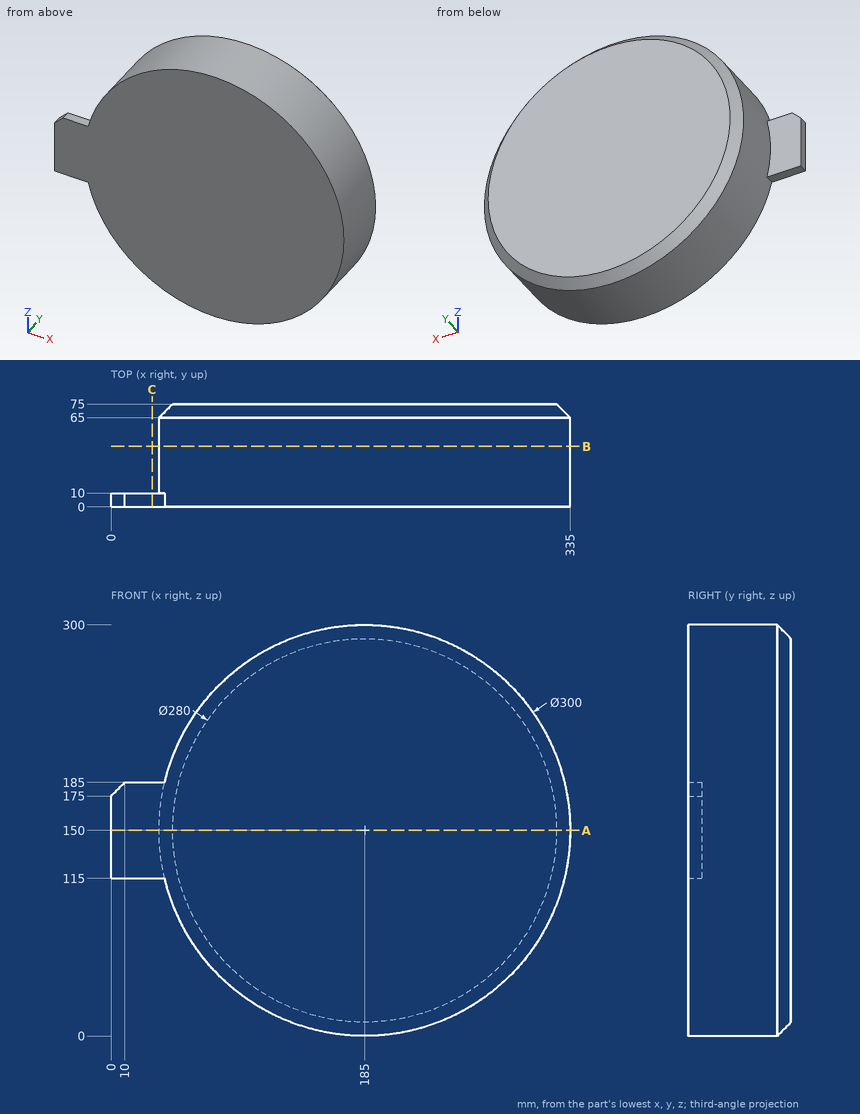
Could you check a few things on this drawing? It's one solid part, dimensions in mm from its lowest x, y, z. Round coordinates to 2 decimals unless told otherwise and drop trailing zeros. Write each loop counter-clockwise with the first axis right and the second up, starting at its lowest first coordinate (ties: lowest second). Pieces come first, ordered by that corner, then holes. Notation, with made-up numbers: (-5, -9) -> (27, -9) arc R20 ccw to (27, 21) -> close; hole circle Ø1 at (-18.5, 47.25). An arc over 180 degrees is marked (long way). Use one line per item in the form item = value. Start each with the question number.
Q1. If I drill on probe 1 along Y at (x, z) = (17, 139); probe 2 along X at (y, z) = (67.5, 143); probe 3 along Z at (x, y) = (68, 34.5), over which ranges is the centre line in solid material (lowest first)? Write a range as [from, to].
Q2. Imagine slicing it at A-A (z = 150). Please give me the cut outline in (x, y).
Q3. I'm going to push flat-ended pins straight in: P1, Ø4, axis at x = 86.5, y = 52.5, coming from the +Z side; P2, Ø6, axis at y = 21, z = 191, coming from the +X side; P3, Ø19.5, axis at x = 15, z = 148, coming from the +Y side. Where does each tip first touch, or does it pass through?
Q4. Imagine slicing it at C-C (x = 30). Please give me the cut outline in (y, z), then the cut area to 3 significant figures.
Q5. Imagine slicing it at B-B (y = 44). Please give me the cut outline in (x, z), then the cut area to 3 significant figures.
Worked out:
q1.probe_1 = [0, 10]
q1.probe_2 = [37.67, 332.33]
q1.probe_3 = [56.13, 243.87]
q2.outline = (0, 0) -> (335, 0) -> (335, 65) -> (325, 75) -> (45, 75) -> (35, 65) -> (35, 10) -> (0, 10) -> close
q3.P1 = 264.84
q3.P2 = 330.11
q3.P3 = 10
q4.outline = (0, 115) -> (10, 115) -> (10, 185) -> (0, 185) -> close
q4.area = 700 mm^2
q5.outline = circle Ø300 at (185, 150)
q5.area = 70,700 mm^2
